Geometry: see drawing. Coordinates: mm, zero at the bounding-box minimum. Round coordinates to 2 decimals unless told otherwise and drop trailing zeros. Order: outer loops, then holes, each group sorted by start corner. A loop starts at its lowest first (then second) coordinate and runs counter-clockwise, first axis right, second up. Notation, with made-up numbers: M -30.75,-13 L 24.25,-13 A20 ccw 24.25,12 Z; hole C -33.75,-38 d6. An arc over 180 degrees is marked long. Answer in a Markdown table with one row per item. Add a question column.
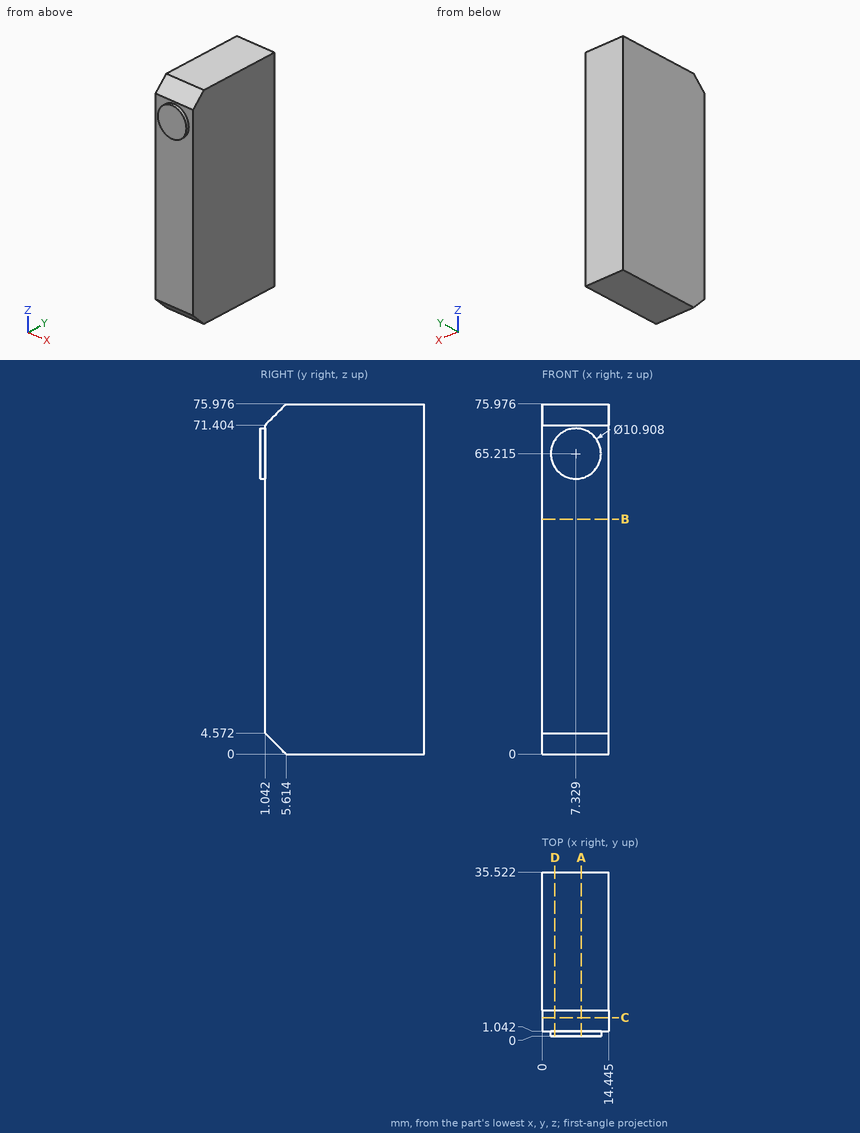
(1) Line query: line 1 (Y direction, x = 11, z = 61); line 2 (Z direction, x = 7.25, y = 3) (1 decimal); line 3 (Y direction, x = 8.75, z = 72). Output: solid intervals per line, ascending. Write a range as from..to.
(2) Cut plane D-D (x = 2.75). Return loops of the section in (y, z) (1 decimal), and give its area (4 significant figures).
(3) Cut plane B-B (z = 51). Return loops of the section in (x, y) (1 decimal).
(4) Cut plane A-A (x = 8.5). Return loops of the section in (y, z) (1 decimal).
(5) Pin query (flat end, axial travel): pin 1 (7 mm diameter, centred on x = 6.5, z = 46.5, fed in from -Y). Return the tip coordinate at first contact, or that it passes through.
(6) Cut plane C-C (y = 4). Return loops of the section in (x, z) (1 decimal).
Answer list:
| question | item | result |
|---|---|---|
| 1 | line 1 | 1.04..35.52 |
| 1 | line 2 | 2.6..73.4 |
| 1 | line 3 | 1.64..35.52 |
| 2 | outline | M 0,62.3 L 1,62.3 L 1,4.6 L 5.6,0 L 35.5,0 L 35.5,76 L 5.6,76 L 1,71.4 L 1,68.2 L 0,68.2 Z |
| 2 | area | 2,605 mm² |
| 3 | outline | M 0,1 L 14.4,1 L 14.4,35.5 L 0,35.5 Z |
| 4 | outline | M 0,59.9 L 1,59.9 L 1,4.6 L 5.6,0 L 35.5,0 L 35.5,76 L 5.6,76 L 1,71.4 L 1,70.5 L 0,70.5 Z |
| 5 | pin 1 | y = 1.04 |
| 6 | outline | M 0,1.6 L 14.4,1.6 L 14.4,74.4 L 0,74.4 Z |
